Verification items for the finished model (mm, model axes). Face numbers are marked on the shaded views. A direction names the side the tool comes from. Give positions to 0.01 mm unless a question says otherwise; leave off trailing zeros. Order: outer loops, then holes, each group sorted by start corner. A loop starts at its lowest first (then second) coordinate and runs counter-clockwise, first axis right, second up.
(1) Gauge pin test, flat ends, axial feed: pin 1 (1.4 mm diameter, centred on x = 44.26, z = -24.82, fed in from -Y); pin 2 (2.5 mm diameter, centred on x = 44.26, z = 34.87, fed in from -Y). Record the tip position at first contact, or that the pin passes through.
(2) Sectioned sample at B-B on x = -23.5. Record the cut outline in (y, z), plus the area to 3 significant figures.
(3) Mould release check, pull along X, two halves, no side actions. Record for the marked faces 1, 2 and 3: pulls with the +X half, pulls with the -X half, needs draft (parallel to the pull), parting line crosses it, or undercut.
(4) Sectioned sample at D-D on y = 5. Record the cut outline in (x, z), plus the area to 3 significant figures.
(5) Sectioned sample at C-C on z = -12. Record the cut outline in (x, y), plus the area to 3 significant figures.
(6) Sectioned sample at A-A on y = 29. Record the cut outline in (x, z), plus the area to 3 significant figures.
(7) Scan lines: L1, parallel to X at y = 17.5, z = 10; L2, parallel to Z at x = -19.5, y = 10.5; L3, parallel to Y at x = -4.5, z = 22. Record each from-to range of solid material in increasing order.
(8) Access from +Z, -Z, +X, -X, +Y, -Y to the whole of each face (thin tool, end or side, straight path). Record for the marked faces 4 and 5.
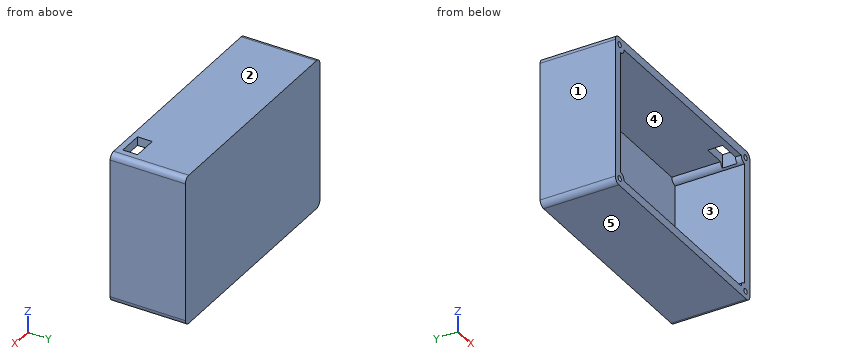
```python
from build123d import *

# Parameters (mm, degrees)
SKETCH1_W           = 99.06
SKETCH1_H           = 66.04
BOSS_EXTRUDE1_DEPTH = 33.02
FILLET1_R           = 2.54
SKETCH3_W           = 91.44
SKETCH3_H           = 58.42
CUT_EXTRUDE1_DEPTH  = 30.48
BOSS_EXTRUDE2_REACH = 74.131
SKETCH4_R           = 1.190625
CUT_EXTRUDE5_DEPTH  = 12.7
CUT_EXTRUDE4_REACH  = 92.093
SKETCH6_W           = 10.795
SKETCH6_H           = 6.477


with BuildPart() as part:
    # Sketch1 → Boss-Extrude1 (new body)
    with BuildSketch(Plane(origin=(0, 0, 0), x_dir=(1, 0, 0), z_dir=(0, 1, 0))):
        with Locations((-2.094797048, -5.024935424)):
            Rectangle(SKETCH1_W, SKETCH1_H)
    extrude(amount=BOSS_EXTRUDE1_DEPTH)

    # Fillet1
    fillet1_edges = [part.edges().sort_by_distance(p)[0] for p in [
        (-51.624797048, 16.51, -27.995064576),
        (47.435202952, 16.51, -27.995064576),
        (47.435202952, 16.51, 38.044935424),
        (-51.624797048, 16.51, 38.044935424),
    ]]
    fillet(fillet1_edges, radius=FILLET1_R)

    # Sketch3 → Cut-Extrude1 (cut)
    with BuildSketch(Plane.XZ):
        with Locations((-2.094797048, 5.024935424)):
            Rectangle(SKETCH3_W, SKETCH3_H)
    extrude(amount=-CUT_EXTRUDE1_DEPTH, mode=Mode.SUBTRACT)

    # Sketch7 → Boss-Extrude2 (add, up to next)
    with BuildSketch(Plane.XZ, mode=Mode.PRIVATE) as boss_extrude2_sk1:
        with BuildLine():
            Line((43.625202952, 34.234935424), (41.085202952, 34.234935424))
            ThreePointArc((41.085202952, 34.234935424), (41.829151728, 32.4388842), (43.625202952, 31.694935424))
            Line((43.625202952, 31.694935424), (43.625202952, 34.234935424))
        make_face()
    boss_extrude2_tool1 = extrude(boss_extrude2_sk1.sketch, amount=-BOSS_EXTRUDE2_REACH, mode=Mode.PRIVATE) - part.part
    # Sketch7 → Boss-Extrude2 (add, up to next)
    with BuildSketch(Plane.XZ, mode=Mode.PRIVATE) as boss_extrude2_sk2:
        with BuildLine():
            Line((-47.814797048, 34.234935424), (-45.274797048, 34.234935424))
            ThreePointArc((-45.274797048, 34.234935424), (-46.018745824, 32.4388842), (-47.814797048, 31.694935424))
            Line((-47.814797048, 31.694935424), (-47.814797048, 34.234935424))
        make_face()
    boss_extrude2_tool2 = extrude(boss_extrude2_sk2.sketch, amount=-BOSS_EXTRUDE2_REACH, mode=Mode.PRIVATE) - part.part
    # Sketch7 → Boss-Extrude2 (add, up to next)
    with BuildSketch(Plane.XZ, mode=Mode.PRIVATE) as boss_extrude2_sk3:
        with BuildLine():
            Line((-47.814797048, -21.645064576), (-47.814797048, -24.185064576))
            Line((-47.814797048, -24.185064576), (-45.274797048, -24.185064576))
            ThreePointArc((-45.274797048, -24.185064576), (-46.018745824, -22.389013351), (-47.814797048, -21.645064576))
        make_face()
    boss_extrude2_tool3 = extrude(boss_extrude2_sk3.sketch, amount=-BOSS_EXTRUDE2_REACH, mode=Mode.PRIVATE) - part.part
    # Sketch7 → Boss-Extrude2 (add, up to next)
    with BuildSketch(Plane.XZ, mode=Mode.PRIVATE) as boss_extrude2_sk4:
        with BuildLine():
            Line((41.085202952, -24.185064576), (43.625202952, -24.185064576))
            Line((43.625202952, -24.185064576), (43.625202952, -21.645064576))
            ThreePointArc((43.625202952, -21.645064576), (41.829151728, -22.389013351), (41.085202952, -24.185064576))
        make_face()
    boss_extrude2_tool4 = extrude(boss_extrude2_sk4.sketch, amount=-BOSS_EXTRUDE2_REACH, mode=Mode.PRIVATE) - part.part
    add(boss_extrude2_tool1.solids().sort_by_distance((42.547193, 0, 33.156926))[0])
    add(boss_extrude2_tool2.solids().sort_by_distance((-46.736788, 0, 33.156926))[0])
    add(boss_extrude2_tool3.solids().sort_by_distance((-46.736788, 0, -23.107055))[0])
    add(boss_extrude2_tool4.solids().sort_by_distance((42.547193, 0, -23.107055))[0])

    # Sketch4 → Cut-Extrude5 (cut)
    with BuildSketch(Plane.XZ):
        with Locations(Location((44.260202952, 34.869935424, 0), (0, 0, 270))):
            Circle(SKETCH4_R)
        with Locations(Location((44.260202952, -24.820064576, 0), (0, 0, 270))):
            Circle(SKETCH4_R)
        with Locations(Location((-48.449797048, 34.869935424, 0), (0, 0, 270))):
            Circle(SKETCH4_R)
        with Locations(Location((-48.449797048, -24.820064576, 0), (0, 0, 270))):
            Circle(SKETCH4_R)
    extrude(amount=-CUT_EXTRUDE5_DEPTH, mode=Mode.SUBTRACT)

    # Sketch6 → Cut-Extrude4 (cut, up to next)
    with BuildSketch(Plane.XY.offset(38.044935424), mode=Mode.PRIVATE) as cut_extrude4_sk1:
        with Locations((36.957702952, 5.7785)):
            Rectangle(SKETCH6_W, SKETCH6_H)
    cut_extrude4_tool1 = extrude(cut_extrude4_sk1.sketch, amount=-CUT_EXTRUDE4_REACH, mode=Mode.PRIVATE) & part.part
    add(cut_extrude4_tool1.solids().sort_by_distance((36.957703, 5.7785, 38.044935))[0], mode=Mode.SUBTRACT)


solid = part.part
```
Ans:
1. pin 1: stops at y = 12.7
1. pin 2: stops at y = 0
2. outline: (0, -28) - (33.02, -28) - (33.02, 38.04) - (0, 38.04) - (0, 34.23) - (30.48, 34.23) - (30.48, -24.19) - (0, -24.19) - close
2. area: 400 mm2
3. face 1: pulls with the -X half
3. face 2: needs draft
3. face 3: undercut
4. outline: (-51.62, -25.46) arc R2.54 ccw to (-49.08, -28) - (44.9, -28) arc R2.54 ccw to (47.44, -25.46) - (47.44, 35.5) arc R2.54 ccw to (44.9, 38.04) - (42.36, 38.04) - (42.36, 32.04) arc R2.54 ccw to (43.63, 31.69) - (43.63, -21.65) arc R2.54 ccw to (41.09, -24.19) - (-45.27, -24.19) arc R2.54 ccw to (-47.81, -21.65) - (-47.81, 31.69) arc R2.54 ccw to (-45.27, 34.23) - (31.56, 34.23) - (31.56, 38.04) - (-49.08, 38.04) arc R2.54 ccw to (-51.62, 35.5) - close; hole circle Ø2.38 at (-48.45, -24.82); hole circle Ø2.38 at (-48.45, 34.87); hole circle Ø2.38 at (44.26, -24.82); hole circle Ø2.38 at (44.26, 34.87)
4. area: 1,150 mm2
5. outline: (-51.62, 0) - (-47.81, 0) - (-47.81, 30.48) - (43.63, 30.48) - (43.63, 0) - (47.44, 0) - (47.44, 33.02) - (-51.62, 33.02) - close
5. area: 484 mm2
6. outline: (-51.62, -25.46) arc R2.54 ccw to (-49.08, -28) - (44.9, -28) arc R2.54 ccw to (47.44, -25.46) - (47.44, 35.5) arc R2.54 ccw to (44.9, 38.04) - (-49.08, 38.04) arc R2.54 ccw to (-51.62, 35.5) - close; hole (-47.81, -21.65) arc R2.54 cw to (-45.27, -24.19) - (41.09, -24.19) arc R2.54 cw to (43.63, -21.65) - (43.63, 31.69) arc R2.54 cw to (41.09, 34.23) - (-45.27, 34.23) arc R2.54 cw to (-47.81, 31.69) - close
6. area: 1,210 mm2
7. L1: x = -51.62 to -47.81, 43.63 to 47.44
7. L2: z = -28 to -24.19, 34.23 to 38.04
7. L3: y = 30.48 to 33.02
8. face 4: -Y
8. face 5: -Z, +X, -X, +Y, -Y
